Drawing for the job (mm, zero at the part's lowest x, y, z). A direction names the side the tool comes from. Give positions to 0.01 mm unless a question says otherwise; leave off trailing zeros. Order: outer loops, then holes, each group sorted by start corner. A loop starts at its lowest first (then second) coordinate and runs counter-clockwise, first axis right, second up. Notation, with made-up numbers: (-22, 7) - (-6, 7) arc R31 ccw to (-6, 38) - close; hole circle Ø2 at (41, -39). An arc over 180 degrees is marked (long way). Use a Markdown table: item, result.
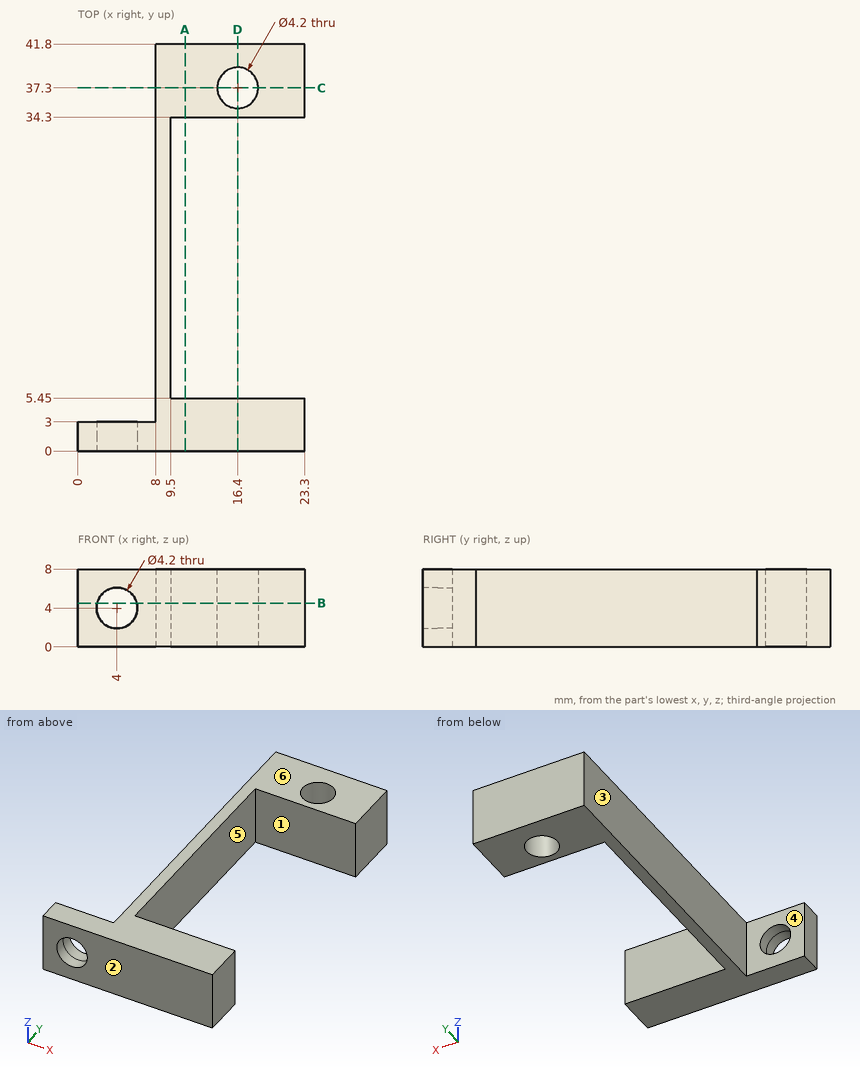
1) Wall check: line 1 (Y direction, x = 16.4, z = 4.25); line 2 (Y direction, x = 11.5, z = 6.5); line 3 (Z direction, x = 4, y = 1.9). Give the ranges that are in metal, low to high. Write a range as from..to.
Computed:
| item | result |
|---|---|
| line 1 | y = 0..5.45, 34.3..35.2, 39.4..41.8 |
| line 2 | y = 0..5.45, 34.3..41.8 |
| line 3 | z = 0..1.9, 6.1..8 |
2) Two-plate mould, pull along Y, no slides. Class the marked faces 4, 5 and 6: +Y half, -Y half, draft (parallel to the pull), parting line (faces both ways), or undercut.
Computed:
| item | result |
|---|---|
| face 4 | +Y half |
| face 5 | undercut |
| face 6 | draft |
3) Tool access for the marked faces 1, 2 and 3: list every direction of +Z, -Z, +X, -X, +Y, -Y with a clear straight run to the whole face (end or side of a thin tool).
Computed:
| item | result |
|---|---|
| face 1 | +Z, -Z, +X |
| face 2 | +Z, -Z, +X, -X, -Y |
| face 3 | +Z, -Z, -X, +Y |
4) Slice it at D-D (x = 16.4). Write the cut outline in (y, z).
Computed:
| item | result |
|---|---|
| outline | (0, 0) - (5.45, 0) - (5.45, 8) - (0, 8) - close; (34.3, 0) - (35.2, 0) - (35.2, 8) - (34.3, 8) - close; (39.4, 0) - (41.8, 0) - (41.8, 8) - (39.4, 8) - close |
5) Slice it at B-B (z = 4.5). Write the cut outline in (x, y), and give its area (3 significant figures).
Computed:
| item | result |
|---|---|
| outline | (0, 0) - (1.96, 0) - (1.96, 3) - (0, 3) - close; (6.04, 0) - (23.3, 0) - (23.3, 5.45) - (9.5, 5.45) - (9.5, 34.3) - (23.3, 34.3) - (23.3, 41.8) - (8, 41.8) - (8, 3) - (6.04, 3) - close; hole circle Ø4.2 at (16.4, 37.3) |
| area | 239 mm² |
6) Slice it at C-C (y = 37.3). Write the cut outline in (x, z), and give its area (3 significant figures).
Computed:
| item | result |
|---|---|
| outline | (8, 0) - (14.3, 0) - (14.3, 8) - (8, 8) - close; (18.5, 0) - (23.3, 0) - (23.3, 8) - (18.5, 8) - close |
| area | 88.8 mm² |
7) Pin check, flat tips, straight feed: P1, Ø1.5, axis at x = 3, z = 2.5, coming from the +Y side; P2, Ø2.5, axis at y = 20, z = 2, coming from the -X side. Stop position of each tip, or through.
Computed:
| item | result |
|---|---|
| P1 | stops at y = 3 |
| P2 | stops at x = 8 |
8) Slice it at A-A (x = 11). Write the cut outline in (y, z).
Computed:
| item | result |
|---|---|
| outline | (0, 0) - (5.45, 0) - (5.45, 8) - (0, 8) - close; (34.3, 0) - (41.8, 0) - (41.8, 8) - (34.3, 8) - close |
